```python
from build123d import *

# Parameters (mm, degrees)
BOSS_EXTRUDE1_DEPTH     = 32.5
SKETCH4_R               = 1.05
BOSS_EXTRUDE2_DEPTH     = 2.5
SKETCH5_R               = 1.05
BOSS_EXTRUDE3_DEPTH     = 3
CUT_EXTRUDE1_DEPTH      = 31.122
BOSS_EXTRUDE4_DEPTH     = 5
BOSS_EXTRUDE6_DEPTH     = 5
CUT_EXTRUDE2_DEPTH      = 6
SKETCH12_W              = 16.4999
SKETCH12_H              = 2
CUT_EXTRUDE4_DEPTH      = 10
CUT_EXTRUDE4_DEPTH_BACK = 23.5


with BuildPart() as part:
    # Sketch2 → Boss-Extrude1 (new body)
    with BuildSketch(Plane(origin=(0, 0, 0), x_dir=(1, 0, 0), z_dir=(0, 1, 0))):
        Polygon((15.061, 0), (15.061, 32), (12.561, 32), (12.561, 2.5), (-12.561, 2.5), (-12.561, 32), (-15.061, 32), (-15.061, 0), align=None)
    extrude(amount=BOSS_EXTRUDE1_DEPTH)

    # Sketch4 → Boss-Extrude2 (add)
    with BuildSketch(Plane.XZ):
        Polygon((-7.5, -6), (7.5, -6), (12.561, -10), (15.061, -10), (15.061, 0), (-15.061, 0), (-15.061, -10), (-12.561, -10), align=None)
        with Locations((-10.2499, -4.95)):
            Circle(SKETCH4_R, mode=Mode.SUBTRACT)
        with Locations((10.2499, -4.95)):
            Circle(SKETCH4_R, mode=Mode.SUBTRACT)
    extrude(amount=BOSS_EXTRUDE2_DEPTH)

    # Sketch5 → Boss-Extrude3 (add)
    with BuildSketch(Plane(origin=(0, 32.5, 0), x_dir=(1, 0, 0), z_dir=(0, 1, 0))):
        Polygon((-15.061, 32), (-10.2499, 32), (-6.25, 26), (6.25, 26), (10.2499, 32), (15.061, 32), (15.061, 0), (-15.061, 0), align=None)
        with Locations((-10.2499, 8.7)):
            Circle(SKETCH5_R, mode=Mode.SUBTRACT)
        with Locations((10.2499, 8.7)):
            Circle(SKETCH5_R, mode=Mode.SUBTRACT)
    extrude(amount=BOSS_EXTRUDE3_DEPTH)

    # Sketch6 → Cut-Extrude1 (cut, through all)
    with BuildSketch(Plane.ZY.offset(15.061)):
        Polygon((-10, 0), (-32, 30.5), (-32, 0), align=None)
    extrude(amount=-CUT_EXTRUDE1_DEPTH, mode=Mode.SUBTRACT)

    # Sketch8 → Boss-Extrude4 (add)
    with BuildSketch(Plane.XY):
        Polygon((0, 76.5), (43.59255168, 16.5), (-43.59255168, 16.5), align=None)
    extrude(amount=BOSS_EXTRUDE4_DEPTH)

    # Sketch9 → Boss-Extrude6 (add)
    with BuildSketch(Plane.XY):
        Polygon((-43.59255168, 16.5), (-58.12340224, -3.5), (58.12340224, -3.5), (43.59255168, 16.5), align=None)
    extrude(amount=BOSS_EXTRUDE6_DEPTH)

    # Sketch10 → Cut-Extrude2 (cut, through all)
    with BuildSketch(Plane(origin=(0, 0, 0), x_dir=(-1, 0, 0), z_dir=(0, 0, -1))):
        Polygon((-29.06170112, -3.5), (-43.59255168, 16.5), (-58.12340224, -3.5), align=None)
        Polygon((58.12340224, -3.5), (43.59255168, 16.5), (29.06170112, -3.5), align=None)
    extrude(amount=-CUT_EXTRUDE2_DEPTH, mode=Mode.SUBTRACT)

    # Sketch12 → Cut-Extrude4 (cut, two sides)
    with BuildSketch(Plane(origin=(0, 0, -26), x_dir=(-1, 0, 0), z_dir=(0, 0, -1))) as cut_extrude4_sk:
        with Locations((0, 33.5)):
            Rectangle(SKETCH12_W, SKETCH12_H)
    extrude(amount=CUT_EXTRUDE4_DEPTH, mode=Mode.SUBTRACT)
    extrude(cut_extrude4_sk.sketch, amount=-CUT_EXTRUDE4_DEPTH_BACK, mode=Mode.SUBTRACT)


solid = part.part
```
Could you check a few things on this model? Use its own coordinates, in mm. A direction names the side the tool comes from. Round coordinates to 2 decimals unless told otherwise and drop trailing zeros. Write each loop counter-clockwise with the first axis right and the second up, starting at its lowest first coordinate (ties: lowest second). Pieces come first, ordered by that corner, then holes.
(1) If I drill on probe 1 along X at (y, z) = (31, -28); probe 2 along X at (y, z) = (-1, -4); probe 3 along X at (y, z) = (34.8, -8.7), over which ranges is the centre line in solid material (lowest first)?
Findings below:
probe 1: x = -15.06 to -12.56, 12.56 to 15.06
probe 2: x = -15.06 to -10.7, -9.8 to 9.8, 10.7 to 15.06
probe 3: x = -15.06 to -11.3, -9.2 to 9.2, 11.3 to 15.06
(2) Suppose I cut it at B-B on z = -24. Write out the boundary of the cut face in (x, y).
Findings below:
outline: (-15.06, 19.41) - (-12.56, 19.41) - (-12.56, 32.5) - (-8.25, 32.5) - (-8.25, 34.5) - (8.25, 34.5) - (8.25, 32.5) - (12.56, 32.5) - (12.56, 19.41) - (15.06, 19.41) - (15.06, 35.5) - (-15.06, 35.5) - close
(3) Which directions (+Z, -Z, +X, -X, +Y, -Y) give clear straight access to the entire face, cutting with the end or side of a thin tool? Please do faces 5 (the face through (0, 35.5, -16)), 6 (the face through (-11.3, -1.2, -4.9)), 7 (the face through (-8.722, 34.312, -29.709)).
Findings below:
face 5: -Z, +X, -X, +Y
face 6: -Y
face 7: -Z, +Y, -Y
(4) Thinking about a two-plate mould opening in X: for faces 1 (the face through (15.061, 20, -13)), 2 (the face through (-13, 34, -32)), 3 (the face through (-36.4, 6.6, 2.5)), 4 (the face through (-10.07, -1.23, -8.03)), which applies, +X half, -X half, draft (parallel to the pull), parting line (faces both ways), or undercut?
Findings below:
face 1: +X half
face 2: draft
face 3: -X half
face 4: undercut
(5) Suppose I cut it at D-D on z = -19. Write out the boundary of the cut face in (x, y).
Findings below:
outline: (-15.06, 12.48) - (-12.56, 12.48) - (-12.56, 32.5) - (-8.25, 32.5) - (-8.25, 34.5) - (8.25, 34.5) - (8.25, 32.5) - (12.56, 32.5) - (12.56, 12.48) - (15.06, 12.48) - (15.06, 35.5) - (-15.06, 35.5) - close
(6) For pin 1 (3 mm diameter, centred on x = 2, y = -1.5, fed in from -Z); pin 2 (0.8 mm diameter, centred on x = -13.5, y = -1.5, fed in from -Z); pin 3 (1.7 mm diameter, centred on x = -10.25, z = -4.95, fed in from -Y), each with a flat end and sliding along its axis, tell me the tip position at first contact or that it passes through.
Findings below:
pin 1: stops at z = -6
pin 2: stops at z = -10
pin 3: stops at y = 32.5
(7) Suppose I cut it at A-A on z = -4.95. Write out the boundary of the cut face in (x, y), and give its area (3 significant figures).
Findings below:
outline: (-15.06, -2.5) - (-11.3, -2.5) - (-11.3, 0) - (-12.56, 0) - (-12.56, 32.5) - (-8.25, 32.5) - (-8.25, 34.5) - (8.25, 34.5) - (8.25, 32.5) - (12.56, 32.5) - (12.56, 0) - (11.3, 0) - (11.3, -2.5) - (15.06, -2.5) - (15.06, 35.5) - (-15.06, 35.5) - close; (-9.2, -2.5) - (9.2, -2.5) - (9.2, 0) - (-9.2, 0) - close
area: 285 mm2
(8) Suppose I cut it at C-C on x = 17. Write out the boundary of the cut face in (y, z).
Findings below:
outline: (-3.5, 0) - (53.1, 0) - (53.1, 5) - (-3.5, 5) - close
